Read the model definition and answer for the solid it produces. Units are mm, in the model's axes. Face numbers are marked on the shaded views. Give positions to 0.01 mm unless a question says otherwise; leave off trailing zeros. Loops run counter-clockwise (first coordinate to the right, second up) from the corner with the lowest first, then second, coordinate; pieces in that order, holes last. Notation, with made-up numbers: (74.5, 30) -> (92.5, 30) arc R32 ccw to (92.5, 63) -> close; hole circle Ø3 at (-15.75, 7). An arc over 180 degrees is marked (long way). One line per item, written item: value. Start each with the question number.
from build123d import *

# Parameters (mm, degrees)
CYLINDER001_R      = 0.85
CYLINDER001_DEPTH  = 50
POLARPATTERN_COUNT = 4


with BuildPart() as part:
    # Cone → Cone (revolve)
    with BuildSketch(Plane.XZ):
        Polygon((0, 0), (10, 0), (13, 25), (0, 25), align=None)
    revolve(axis=Axis((0, 0, 0), (0, 0, 1)))

    # Cylinder001 → Cylinder001 (cut)
    with BuildSketch(Plane(origin=(4.5, 4.5, 0), x_dir=(1, 0, 0), z_dir=(0, 0, 1))):
        Circle(CYLINDER001_R)
    cylinder001 = extrude(amount=CYLINDER001_DEPTH, mode=Mode.SUBTRACT)

    # PolarPattern: Cylinder001 ×4 about axis
    polarpattern_axis = Axis((0, 0, 0), (0, 0, 1))
    for i in range(1, POLARPATTERN_COUNT):
        add(cylinder001.rotate(polarpattern_axis, i * 360 / POLARPATTERN_COUNT), mode=Mode.SUBTRACT)


solid = part.part
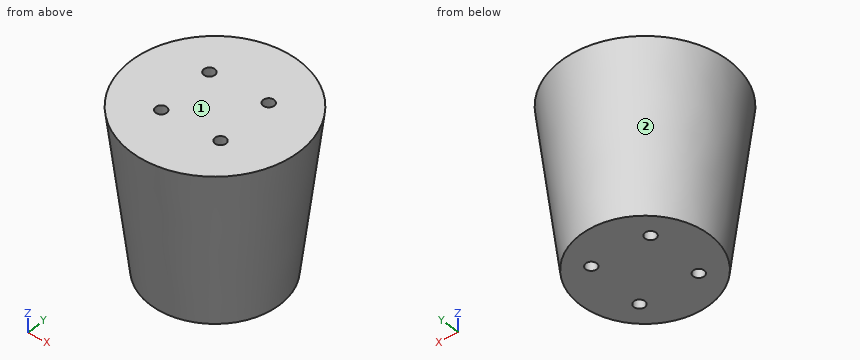
Item 1: Section A-A, the plane z = 13.5 is taken. Determine the outline of the cut face in (x, y), plus the area to 3 significant figures.
Item 2: Section B-B, the plane x = 0 is taken. Determine the outline of the cut face in (y, z).
Item 3: Flat-ended cylindrical pins translate along their axes: pin 1 (12 mm diameter, centred on x = 8.5, z = 20, fed in from -Y); pin 2 (2 mm diameter, centred on x = -4, z = 17, fed in from +Y); pin 3 (5 mm diameter, centred on y = -10.5, z = 2.5, fed in from +X). Find the tip coordinate at first contact, or state that the pin passes through.
Item 4: Section C-C, the plane z = 5 is taken. Determine the outline of the cut face in (x, y), plus the area to 3 significant figures.
Item 5: Determine the mould class of the marked faces 1 and 2 for opening direction Y: pulls with the +Y half, pulls with the -Y half, needs draft (parallel to the pull), parting line crosses it, or undercut.
Item 6: Consider L1, parallel to X at y = -4.25, z = 18.75; L2, parallel to X at y = 4.5, z = 17.75; L3, parallel to Y at x = 4.5, z = 6.5. Determine where each line is inside the solid, lowest interval first. Write a range as [from, to].
Computed values:
1. outline: circle Ø23.24 at (0, 0); hole circle Ø1.7 at (-4.5, -4.5); hole circle Ø1.7 at (-4.5, 4.5); hole circle Ø1.7 at (4.5, -4.5); hole circle Ø1.7 at (4.5, 4.5)
1. area: 415 mm²
2. outline: (-13, 25) -> (-10, 0) -> (10, 0) -> (13, 25) -> close
3. pin 1: y = -12.33
3. pin 2: y = 11.69
3. pin 3: x = 6.52
4. outline: circle Ø21.2 at (0, 0); hole circle Ø1.7 at (-4.5, -4.5); hole circle Ø1.7 at (-4.5, 4.5); hole circle Ø1.7 at (4.5, -4.5); hole circle Ø1.7 at (4.5, 4.5)
4. area: 344 mm²
5. face 1: needs draft
5. face 2: parting line crosses it
6. L1: [-11.49, -5.31], [-3.69, 3.69], [5.31, 11.49]
6. L2: [-11.26, -5.35], [-3.65, 3.65], [5.35, 11.26]
6. L3: [-9.8, -5.35], [-3.65, 3.65], [5.35, 9.8]
